```python
from build123d import *

# Parameters (mm, degrees)
ESBO_O1_R                = 4
RESSALTO_EXTRUS_O1_DEPTH = 101.7
CHANFRO1_SIZE            = 1
ESBO_O2_W                = 8.479156614
ESBO_O2_H                = 1.5
CORTE_EXTRUS_O1_DEPTH    = 2


with BuildPart() as part:
    # BodySke → BaseBody (revolve)
    with BuildSketch(Plane.XY, mode=Mode.PRIVATE) as basebody_sk:
        Polygon((0, 0), (0, 2.4455), (0.320140724, 3), (11, 3), (12, 2), (12, 0), align=None)
    revolve(basebody_sk.sketch.rotate(Axis((-12.7, 0, 0), (1, 0, 0)), 90), axis=Axis((-12.7, 0, 0), (1, 0, 0)))

    # Esboço1 → Ressalto-extrusão1 (add)
    with BuildSketch(Plane(origin=(0, 0, 0), x_dir=(0, 0, -1), z_dir=(1, 0, 0))):
        Circle(ESBO_O1_R)
    extrude(amount=-RESSALTO_EXTRUS_O1_DEPTH)

    # Chanfro1
    chanfro1_edges = [part.edges().sort_by_distance(p)[0] for p in [
        (0, 0, 4),
    ]]
    chamfer(chanfro1_edges, length=CHANFRO1_SIZE)

    # Esboço2 → Corte-extrusão1 (cut)
    with BuildSketch(Plane.ZY.offset(101.7)):
        Rectangle(ESBO_O2_W, ESBO_O2_H)
    extrude(amount=-CORTE_EXTRUS_O1_DEPTH, mode=Mode.SUBTRACT)


solid = part.part
```
Verification items for the finished model (mm, model axes). A direction names the side the tool comes from. Coordinates: 2 decimals unless noted, no trailing zeros. Write each loop counter-clockwise with the first axis right and the second up, starting at its lowest first coordinate (ties: lowest second). Pieces come first, ordered by that corner, then holes. Notation, with made-up numbers: M -22,-15.5 L -8,-15.5 A17 cw -8,3.5 Z; hole C 44,-26.75 d9. An arc over 180 degrees is marked long. One line per item, written item: value.
Item 1: Section check A-A, the plane z = 0. Record the boundary of the cut face in (x, y).
Check sheet entries:
outline: M -101.7,-4 L -1,-4 L 0,-3 L 0,-2.45 L 0.32,-3 L 11,-3 L 12,-2 L 12,2 L 11,3 L 0.32,3 L 0,2.45 L 0,3 L -1,4 L -101.7,4 L -101.7,0.75 L -99.7,0.75 L -99.7,-0.75 L -101.7,-0.75 Z
Item 2: Access from +Z, -Z, +X, -X, +Y, -Y to the whole of each face (thin tool, end or side, straight path). Record for faces 4 (the flat face through (-101, 0.75, 0)), 5 (the flat face through (12, 0, 0)).
Check sheet entries:
face 4: +Z, -Z, -X
face 5: +Z, -Z, +X, +Y, -Y
Item 3: Mould release check, pull along Y, two halves, no side actions. Record for faces 1 (the flat face through (-101.7, 2, 0)), 2 (the flat face through (-101, -0.75, 0)), 3 (the cylindrical face through (5.73, -0.9, 2.86)): pulls with the +Y half, pulls with the -Y half, needs draft (parallel to the pull), parting line crosses it, or undercut.
Check sheet entries:
face 1: needs draft
face 2: undercut
face 3: parting line crosses it
Item 4: Scan lines: line 1 along X through (y, z) = (0.25, 1); line 2 along Z through (x, y) = (-80.5, -1.25); line 3 along X through (y, z) = (2.25, 0). Record each from-to range of solid material in increasing order.
Check sheet entries:
line 1: x = -99.7 to 12
line 2: z = -3.8 to 3.8
line 3: x = -101.7 to 11.75
Item 5: Gauge pin test, flat ends, axial feed: pin 1 Ø0.6 at (x, z) = (-101, 1.5) entering from +Y; pin 2 Ø2 at (x, z) = (-28.5, 2.5) entering from +Y; pin 3 Ø3 at (x, z) = (-70.5, -2) entering from +Y. Record the tip position at first contact, or that the pin passes through.
Check sheet entries:
pin 1: stops at y = 3.82
pin 2: stops at y = 3.71
pin 3: stops at y = 3.97
Item 6: Section check B-B, the plane x = -2.5. Record the boundary of the cut face in (y, z), plus the area to 3 significant figures.
Check sheet entries:
outline: C 0,0 d8
area: 50.3 mm^2
